from build123d import *

# Parameters (mm, degrees)
CROQUIS1_W              = 59.5
CROQUIS1_H              = 34
CROQUIS1_W_2            = 56.5
CROQUIS1_H_2            = 31
EXTRUIR_L_MINA1_DEPTH   = 19
CROQUIS2_W              = 59.5
CROQUIS2_H              = 34
SALIENTE_EXTRUIR1_DEPTH = 2
SALIENTE_EXTRUIR3_DEPTH = 34
CROQUIS5_W              = 59.5
CROQUIS5_H              = 1.5
SALIENTE_EXTRUIR4_DEPTH = 3.5
CROQUIS6_W              = 5
CROQUIS6_H              = 5
CORTAR_EXTRUIR1_DEPTH   = 3.5
CROQUIS7_R              = 1.75
CORTAR_EXTRUIR2_DEPTH   = 3.5
EXTRUIR_L_MINA2_DEPTH   = 3


with BuildPart() as part:
    # Croquis1 → Extruir-Lámina1 (new body)
    with BuildSketch(Plane.XY):
        Rectangle(CROQUIS1_W, CROQUIS1_H)
        Rectangle(CROQUIS1_W_2, CROQUIS1_H_2, mode=Mode.SUBTRACT)
    extrude(amount=EXTRUIR_L_MINA1_DEPTH)

    # Croquis2 → Saliente-Extruir1 (add)
    with BuildSketch(Plane(origin=(0, 0, 0), x_dir=(-1, 0, 0), z_dir=(0, 0, -1))):
        Rectangle(CROQUIS2_W, CROQUIS2_H)
    extrude(amount=SALIENTE_EXTRUIR1_DEPTH)

    # Croquis4 → Saliente-Extruir3 (add)
    with BuildSketch(Plane(origin=(0, 17, 0), x_dir=(1, 0, 0), z_dir=(0, 1, 0))):
        Polygon((-29.75, -19), (-29.75, -22.5), (-24.75, -22.5), (-24.75, -21), (-27.75, -21), (-27.75, -19), align=None)
        Polygon((27.75, -21), (27.75, -19), (29.75, -19), (29.75, -22.5), (24.75, -22.5), (24.75, -21), align=None)
    extrude(amount=-SALIENTE_EXTRUIR3_DEPTH)

    # Croquis5 → Saliente-Extruir4 (add)
    with BuildSketch(Plane.XY.offset(19)):
        with Locations((0, -16.25)):
            Rectangle(CROQUIS5_W, CROQUIS5_H)
    extrude(amount=SALIENTE_EXTRUIR4_DEPTH)

    # Croquis6 → Cortar-Extruir1 (cut)
    with BuildSketch(Plane.XY):
        with Locations((-25.75, -13)):
            Rectangle(CROQUIS6_W, CROQUIS6_H)
    extrude(amount=-CORTAR_EXTRUIR1_DEPTH, mode=Mode.SUBTRACT)

    # Croquis7 → Cortar-Extruir2 (cut)
    with BuildSketch(Plane(origin=(0, 0, -2), x_dir=(-1, 0, 0), z_dir=(0, 0, -1))):
        with Locations((20.75, 12.11)):
            Circle(CROQUIS7_R)
        with Locations((20.75, -9.14)):
            Circle(CROQUIS7_R)
        with Locations((-24.25, -9.14)):
            Circle(CROQUIS7_R)
        with Locations((-24.25, 12.11)):
            Circle(CROQUIS7_R)
    extrude(amount=-CORTAR_EXTRUIR2_DEPTH, mode=Mode.SUBTRACT)

    # Croquis8 → Extruir-Lámina2 (add)
    with BuildSketch(Plane.XY):
        Polygon((-15.784787685, 12.11), (-18.267393842, 16.41), (-23.232606158, 16.41), (-25.715212315, 12.11), (-23.232606158, 7.81), (-18.267393842, 7.81), align=None)
        Polygon((-17.516838493, 12.11), (-19.133419246, 14.91), (-22.366580754, 14.91), (-23.983161507, 12.11), (-22.366580754, 9.31), (-19.133419246, 9.31), align=None, mode=Mode.SUBTRACT)
        Polygon((29.215212315, 12.11), (26.732606158, 16.41), (21.767393842, 16.41), (19.284787685, 12.11), (21.767393842, 7.81), (26.732606158, 7.81), align=None)
        Polygon((27.483161507, 12.11), (25.866580754, 14.91), (22.633419246, 14.91), (21.016838493, 12.11), (22.633419246, 9.31), (25.866580754, 9.31), align=None, mode=Mode.SUBTRACT)
        Polygon((-15.784787685, -9.14), (-18.267393842, -4.84), (-23.232606158, -4.84), (-25.715212315, -9.14), (-23.232606158, -13.44), (-18.267393842, -13.44), align=None)
        Polygon((-17.516838493, -9.14), (-19.133419246, -6.34), (-22.366580754, -6.34), (-23.983161507, -9.14), (-22.366580754, -11.94), (-19.133419246, -11.94), align=None, mode=Mode.SUBTRACT)
        Polygon((29.215212315, -9.14), (26.732606158, -4.84), (21.767393842, -4.84), (19.284787685, -9.14), (21.767393842, -13.44), (26.732606158, -13.44), align=None)
        Polygon((27.483161507, -9.14), (25.866580754, -6.34), (22.633419246, -6.34), (21.016838493, -9.14), (22.633419246, -11.94), (25.866580754, -11.94), align=None, mode=Mode.SUBTRACT)
    extrude(amount=EXTRUIR_L_MINA2_DEPTH)


solid = part.part
The listing builds one solid part. Answer for the finished solid, in the listing's coordinates (mm). A direction names the side the tool comes from. Coordinates: 2 decimals unless noted, no trailing zeros. Write each loop counter-clockwise with the first axis right and the second up, starting at its lowest first coordinate (ties: lowest second). Pieces come first, ordered by that corner, then holes. Notation, with made-up numbers: (-25, -8) - (3, -8) arc R16 cw to (3, 18) - close; hole circle Ø2 at (78.25, 84). An arc over 180 degrees is marked (long way). Answer as CSV lines item,"result".
1. Find section B-B (x = -20.75). Give the number of separate pieces and of enclosed holes in the cut face, plus the area to 3 significant figures.
Computed values:
separate pieces,"3"
enclosed holes,"0"
area,"132 mm²"
2. Straight lines are drawn through the part: line 1 (Y direction, x = -20.75, z = -1.4); line 2 (X direction, y = 4.5, z = 6); line 3 (Y direction, x = -16, z = 8.25). For each, find the intervals that lie inside material, in ascending order. Write a range as [from, to].
Computed values:
line 1,"y = [-17, -10.89], [-7.39, 10.36], [13.86, 17]"
line 2,"x = [-29.75, -28.25], [28.25, 29.75]"
line 3,"y = [-17, -15.5], [15.5, 17]"
3. Find section A-A (z = 16.25). Give the vertices of the cut face in (x, y), plus the area to 4 significant figures.
Computed values:
outline,"(-29.75, -17) - (29.75, -17) - (29.75, 17) - (-29.75, 17) - close; hole (-28.25, -15.5) - (28.25, -15.5) - (28.25, 15.5) - (-28.25, 15.5) - close"
area,"271.5 mm²"
4. A tool of negligible diameter and unlimited length cuts with its end or side. For faces 1 (the flat face through (-26, 1, 21)), 2 (the flat face through (-23.25, -13, -1)), 3 (the flat face through (-16.75, 13.78, 1.48)), 4 (the flat face through (-24.72, 13.83, 1.48)), from which of +Z, -Z, +X, -X, +Y, -Y can it reach the whole face along a straight path? Write none if from no direction.
Computed values:
face 1,"+Y"
face 2,"-Z"
face 3,"+Z"
face 4,"none"
5. Given P1, Ø2.5, axis at x = 22.5, y = 12.5, coming from the +Z side, flat-ended and moving along its own axis, determine where the tip first touches the part or whether it passes through.
Computed values:
P1,"stops at z = 3"
6. Find section C-C (y = 2). Give the vertices of the cut face in (x, z).
Computed values:
outline,"(-29.75, -2) - (29.75, -2) - (29.75, 22.5) - (24.75, 22.5) - (24.75, 21) - (27.75, 21) - (27.75, 19) - (28.25, 19) - (28.25, 0) - (-28.25, 0) - (-28.25, 19) - (-27.75, 19) - (-27.75, 21) - (-24.75, 21) - (-24.75, 22.5) - (-29.75, 22.5) - close"
